from build123d import *

# Parameters (mm, degrees)
SKETCH2_R           = 3.5
BOSS_EXTRUDE1_DEPTH = 1
SKETCH4_R           = 0.4
CUT_EXTRUDE2_DEPTH  = 6.049752469
CUT_EXTRUDE3_DEPTH  = 6.049752469
CIRPATTERN1_COUNT   = 4


with BuildPart() as part:
    # Sketch2 → Boss-Extrude1 (new body)
    with BuildSketch(Plane.XY):
        Circle(SKETCH2_R)
    extrude(amount=BOSS_EXTRUDE1_DEPTH)

    # Sketch4 → Cut-Extrude2 (cut, through all)
    with BuildSketch(Plane.XY.offset(1)):
        Circle(SKETCH4_R)
    extrude(amount=-CUT_EXTRUDE2_DEPTH, mode=Mode.SUBTRACT)

    # Sketch5 → Cut-Extrude3 (cut, through all)
    with BuildSketch(Plane.XY.offset(1)):
        with BuildLine():
            Line((-1.060660172, -1.060660172), (-1.838477631, -1.838477631))
            ThreePointArc((-1.838477631, -1.838477631), (-0.994976924, -2.402086785), (0, -2.6))
            Line((0, -2.6), (0, -1.5))
            ThreePointArc((0, -1.5), (-0.574025149, -1.385819299), (-1.060660172, -1.060660172))
        make_face()
    cut_extrude3 = extrude(amount=-CUT_EXTRUDE3_DEPTH, mode=Mode.SUBTRACT)

    # CirPattern1: Cut-Extrude3 ×4 about axis
    cirpattern1_axis = Axis((0, 0, 1), (0, 0, 1))
    for i in range(1, CIRPATTERN1_COUNT):
        add(cut_extrude3.rotate(cirpattern1_axis, i * 360 / CIRPATTERN1_COUNT), mode=Mode.SUBTRACT)


solid = part.part
Source: CAD feature listing. Evaluate the final solid. Frame: model axes, mm. A direction names the side the tool comes from. Round coordinates to 2 decimals unless told otherwise and drop trailing zeros. Loops run counter-clockwise (first coordinate to the right, second up) from the corner with the lowest first, then second, coordinate; pieces in that order, holes last.
Q1. Mould query, pull axis Y, two halves, no side actions, for faces 3 (the face through (1, 0, 0)), 4 (the face through (3.233, -1.341, 0.493)), 5 (the face through (2.1, 0, 0.5)). Classes: pulls with the +Y half, pulls with the -Y half, needs draft (parallel to the pull), parting line crosses it, or undercut.
Q2. Section B-B, the plane y = -0.25. Return loops of the section in (x, z).
Q3. Section A-A, the plane z = 0.55. Return loops of the section in (x, y), plus the area to 3 significant figures.
Q4. Section D-D, the plane x = -1.25. Return loops of the section in (y, z), plus the area to 3 significant figures.
Q5. First-contact query: P1, Ø1.5, axis at x = -0.5, y = -1, coming from the -Z side. Flat tip, straight axial feed; report the tip coordinate or a pass-through.
Q6. Access query for faces 1 (the face through (-1.389, 0.566, 0.507)), 2 (the face through (1, 0, 1)). Directions: +Z, -Z, +X, -X, +Y, -Y. A direction counts if a zero-diameter tool reaches every point of the face in a straight line with its end or side. Return the directions, or none.
Q7. Section C-C, the plane x = 2.5. Return loops of the section in (y, z), plus the area to 3 significant figures.
Q8. Ray query, line 1 (Y direction, x = -1.75, z = 0.45); line 2 (X direction, y = 0.25, z = 0.8); line 3 (X direction, y = -1, z = 0.95). Return the intervals inside material, ascending.
Solutions:
1. face 3: needs draft
1. face 4: parting line crosses it
1. face 5: undercut
2. outline: (-3.49, 0) - (-0.31, 0) - (-0.31, 1) - (-3.49, 1) - close; (0.31, 0) - (1.48, 0) - (1.48, 1) - (0.31, 1) - close; (2.59, 0) - (3.49, 0) - (3.49, 1) - (2.59, 1) - close
3. outline: circle Ø7 at (0, 0); hole (-2.6, 0) - (-1.5, 0) arc R1.5 cw to (-1.06, 1.06) - (-1.84, 1.84) arc R2.6 ccw to start; hole (-1.84, -1.84) arc R2.6 ccw to (0, -2.6) - (0, -1.5) arc R1.5 cw to (-1.06, -1.06) - close; hole circle Ø0.8 at (0, 0); hole (0, 1.5) arc R1.5 cw to (1.06, 1.06) - (1.84, 1.84) arc R2.6 ccw to (0, 2.6) - close; hole (1.06, -1.06) - (1.84, -1.84) arc R2.6 ccw to (2.6, 0) - (1.5, 0) arc R1.5 cw to start
3. area: 30.9 mm2
4. outline: (-3.27, 0) - (-2.28, 0) - (-2.28, 1) - (-3.27, 1) - close; (-1.25, 0) - (0.83, 0) - (0.83, 1) - (-1.25, 1) - close; (1.25, 0) - (3.27, 0) - (3.27, 1) - (1.25, 1) - close
4. area: 5.09 mm2
5. P1: stops at z = 0
6. face 1: +Z, -Z
6. face 2: +Z, +X, -X, +Y, -Y
7. outline: (-2.45, 0) - (-0.71, 0) - (-0.71, 1) - (-2.45, 1) - close; (0, 0) - (2.45, 0) - (2.45, 1) - (0, 1) - close
7. area: 4.18 mm2
8. line 1: y = -3.03 to -1.92, -1.75 to 0, 1.75 to 3.03
8. line 2: x = -3.49 to -2.59, -1.48 to -0.31, 0.31 to 3.49
8. line 3: x = -3.35 to 1.12, 2.4 to 3.35
